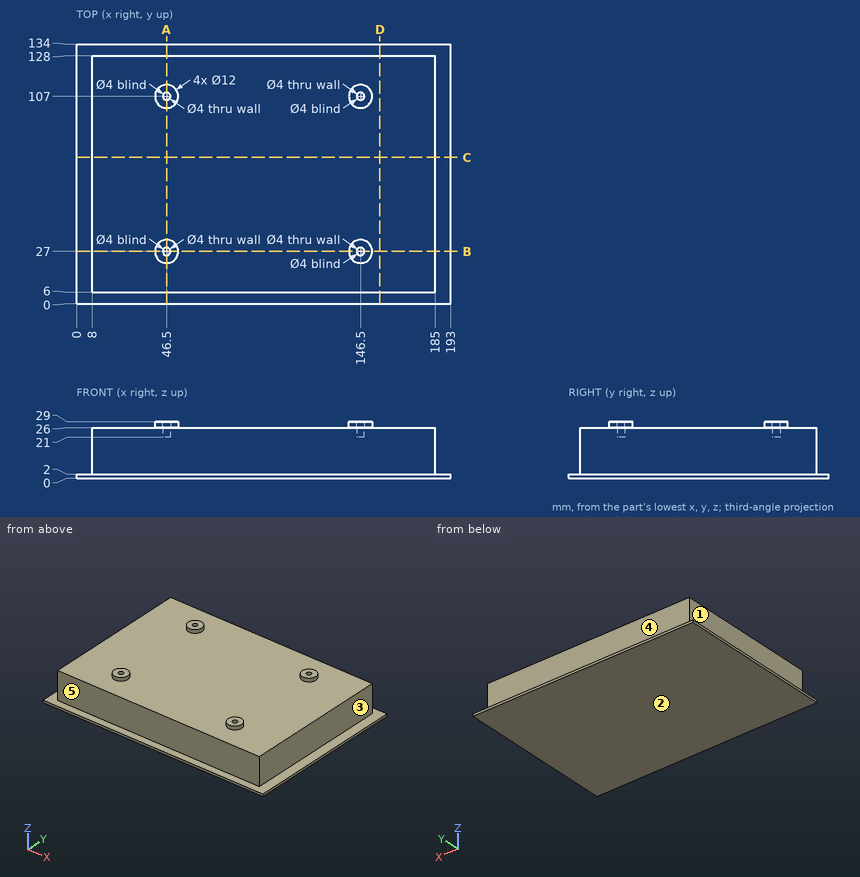
Can you work these out from the drawing? Everything is in mm from the part's minimum corner. A direction names the side the tool comes from. Give positions to 0.01 mm unless a question says otherwise; leave off trailing zeros. Order: outer loops, then holes, each group sorted by start corner. A loop starts at its lowest first (then second) coordinate and runs counter-clockwise, first axis right, second up. Notation, with made-up numbers: M 19,-33.5 L 31,-33.5 A7 ccw 31,-26.5 Z; hole C -35,19.5 d11. An arc over 180 degrees is marked long. One line per question, with ' | ' between items.
1. I want a section at D-D (x = 156.5). List the corners of the cut face in (y, z) for me.
Results:
outline: M 0,0 L 134,0 L 134,2 L 128,2 L 128,26 L 6,26 L 6,2 L 0,2 Z
2. I want a section at B-B (y = 27). List the corners of the cut face in (x, z) for me, and give its area (3 significant figures).
Results:
outline: M 0,0 L 193,0 L 193,2 L 185,2 L 185,26 L 152.5,26 L 152.5,29 L 148.5,29 L 148.5,21 L 144.5,21 L 144.5,29 L 140.5,29 L 140.5,26 L 52.5,26 L 52.5,29 L 48.5,29 L 48.5,21 L 44.5,21 L 44.5,29 L 40.5,29 L 40.5,26 L 8,26 L 8,2 L 0,2 Z | area: 4,640 mm²
3. I want a section at A-A (x = 46.5). List the corners of the cut face in (y, z) for me.
Results:
outline: M 0,0 L 134,0 L 134,2 L 128,2 L 128,26 L 113,26 L 113,29 L 109,29 L 109,21 L 105,21 L 105,29 L 101,29 L 101,26 L 33,26 L 33,29 L 29,29 L 29,21 L 25,21 L 25,29 L 21,29 L 21,26 L 6,26 L 6,2 L 0,2 Z
4. I'm going to push flat-ended pins straight in: pin 1 (4 mm diameter, centred on y = 34.5, z = 18, fed in from +X); pin 2 (7 mm diameter, centred on y = 64, z = 13.5, fed in from -X); pin 3 (5 mm diameter, centred on x = 167.5, z = 23, fed in from -Y). Where does each tip first touch, or does it pass through?
Results:
pin 1: x = 185 | pin 2: x = 8 | pin 3: y = 6
5. For the marked faces 1, 2, 3, 4 and 5, which set-ups out of +Z, -Z, +X, -X, +Y, -Y let a thin tool reach every point of the face, with its end or its side?
Results:
face 1: +Z, -X, +Y, -Y | face 2: -Z, +X, -X, +Y, -Y | face 3: +Z, +X, +Y, -Y | face 4: +Z, +X, -X, +Y | face 5: +Z, +X, -X, -Y
6. If I drill on line 1 (X direction, y = 27, z = 22.6); line 2 (Y direction, x = 46.5, z = 27.1); line 3 (Y direction, x = 146.5, z = 22.6), over which ranges is the centre line in solid material (lowest first)?
Results:
line 1: 8 to 44.5, 48.5 to 144.5, 148.5 to 185 | line 2: 21 to 25, 29 to 33, 101 to 105, 109 to 113 | line 3: 6 to 25, 29 to 105, 109 to 128
7. I want a section at C-C (y = 75.5). List the corners of the cut face in (x, z) for me.
Results:
outline: M 0,0 L 193,0 L 193,2 L 185,2 L 185,26 L 8,26 L 8,2 L 0,2 Z
